Read the model definition and answer for the solid it produces. Units are mm, in the model's axes. A direction names the side the tool comes from. Give positions to 0.01 mm unless a question says otherwise; leave off trailing zeros. Order: outer loops, then holes, each group sorted by start corner. A loop starts at its lowest first (then second) coordinate and runs counter-clockwise, first axis right, second up.
```python
from build123d import *

# Parameters (mm, degrees)
CUT_EXTRUDE1_DEPTH = 4
CUT_EXTRUDE2_DEPTH = 5.5


with BuildPart() as part:
    # Sketch1 → Revolve1 (revolve)
    with BuildSketch(Plane.XY, mode=Mode.PRIVATE) as revolve1_sk:
        Polygon((-68.909512761, 0), (-68.909512761, 11.5), (-67.909512761, 12.5), (-26.409512761, 12.5), (-26.409512761, 16.5), (-25.409512761, 17.5), (8.590487239, 17.5), (8.590487239, 23.5), (9.590487239, 24.5), (30.090487239, 24.5), (31.090487239, 23.5), (31.090487239, 17.5), (100.090487239, 17.5), (101.090487239, 16.5), (101.090487239, 12.5), (117.090487239, 12.5), (118.090487239, 11.5), (118.090487239, 0), align=None)
    revolve(revolve1_sk.sketch.rotate(Axis((-92.22737819, 0, 0), (1, 0, 0)), 90), axis=Axis((-92.22737819, 0, 0), (1, 0, 0)))

    # Sketch2 → Cut-Extrude1 (cut)
    with BuildSketch(Plane(origin=(0, 17.5, 0), x_dir=(1, 0, 0), z_dir=(0, 1, 0))):
        with BuildLine():
            Line((-20.909512761, 4), (4.090487239, 4))
            ThreePointArc((4.090487239, 4), (8.090487239, 0), (4.090487239, -4))
            Line((4.090487239, -4), (-20.909512761, -4))
            ThreePointArc((-20.909512761, -4), (-24.909512761, 0), (-20.909512761, 4))
        make_face()
    extrude(amount=-CUT_EXTRUDE1_DEPTH, mode=Mode.SUBTRACT)

    # Sketch3 → Cut-Extrude2 (cut)
    with BuildSketch(Plane(origin=(0, 17.5, 0), x_dir=(1, 0, 0), z_dir=(0, 1, 0))):
        with BuildLine():
            Line((40.590487239, 7), (90.590487239, 7))
            ThreePointArc((90.590487239, 7), (97.590487239, 0), (90.590487239, -7))
            Line((90.590487239, -7), (40.590487239, -7))
            ThreePointArc((40.590487239, -7), (33.590487239, 0), (40.590487239, 7))
        make_face()
    extrude(amount=-CUT_EXTRUDE2_DEPTH, mode=Mode.SUBTRACT)


solid = part.part
```
1) For a pull along Z with two mould halves and no side action, classify faces 1 (the face through (19.98, -7.36, 23.37)), 2 (the face through (31.09, -18, 0)), 3 (the face through (-8, 13.5, 0)) as released by +Z, released by -Z, zero draft, split by the parting line, or undercut.
Final values:
face 1: split by the parting line
face 2: zero draft
face 3: undercut
2) Given pin 1 (8 mm diameter, centred on x = 51, y = 15, fed in from +Z); pin 2 (4.5 mm diameter, centred on x = 73, y = 15, fed in from +Z); pin 3 (1.5 mm diameter, centred on x = 61, y = 14, fed in from -Z), each flat-ended and moving along its own axis, determine where each tip first touches the part or whether it passes through.
Final values:
pin 1: stops at z = 13.61
pin 2: stops at z = 11.99
pin 3: stops at z = -11.43
3) The part is cut by section D-D on x = -51. Determine the outline of the cut face in (y, z), and give its area (3 significant figures).
Final values:
outline: circle Ø25 at (0, 0)
area: 491 mm2
4) The part is cut by section B-B on x = 12. Determine the outline of the cut face in (y, z), and give its area (3 significant figures).
Final values:
outline: circle Ø49 at (0, 0)
area: 1,890 mm2
5) Consider L1, parallel to Y at x = 109, z = -0.5; L2, parallel to X at y = -13, z = -0.5; L3, parallel to X at y = -6.5, z = 19.5. Determine where each line is inside the solid, lowest interval first.
Final values:
L1: y = -12.49 to 12.49
L2: x = -26.41 to 101.09
L3: x = 8.59 to 31.09
6) A tool of negligible diameter and unlimited length cuts with its end or side. For faces 4 (the face through (-8.172, -14.756, 9.408)), 5 (the face through (-68.91, 0, 0)), 6 (the face through (101.09, -3.7, -12.3)), 7 (the face through (-9, 15, -4)), from which of +Z, -Z, +X, -X, +Y, -Y can it reach the whole face along a straight path? Write none if from no direction.
Final values:
face 4: -X
face 5: +Z, -Z, -X, +Y, -Y
face 6: +X
face 7: +Y
7) The part is cut by section C-C on x = 52. Determine the outline of the cut face in (y, z), and give its area (3 significant figures).
Final values:
outline: (12, -7) - (12, 7) - (16.04, 7) arc R17.5 ccw (long way) to (16.04, -7) - close
area: 892 mm2
